Geometry check sheet. Reference: the model listing, model coordinates, mm. A direction names the side the tool comes from. Round coordinates to 2 decimals unless told otherwise and drop trailing zeros. Loops run counter-clockwise (first coordinate to the right, second up) from the corner with the lowest first, then second, coordinate; pieces in that order, holes last. Notation, with made-up numbers: (-16, -18.5) - (35, -18.5) arc R23 cw to (35, 19.5) - close; hole circle Ø11 at (73, 52.25). An arc over 180 degrees is marked (long way). Write item = value, one per line.
```python
from build123d import *

# Parameters (mm, degrees)
BOSS_EXTRU_1_DEPTH      = 200
ENL_V_MAT_EXTRU_1_DEPTH = 274.130005675
SYM_TRIE2_COPY_1_DEPTH  = 200
SYM_TRIE2_COPY_2_DEPTH  = 274.130005675
SYM_TRIE2_COPY_3_DEPTH  = 274.130005675
INTERSECT1_START        = -110
INTERSECT1_DEPTH        = 220


# Read off the part's stored shape, not the designer's step: Intersect1
with BuildPart() as part:
    # Esquisse1 → Boss.-Extru.1 (new body)
    with BuildSketch(Plane.XY):
        Polygon((0, 0), (0, 150), (110, 150), (110, 100), (102.516685226, 87), (102.516685226, 77), (110, 64), (110, 14), (71, 0), align=None)
    boss_extru_1 = extrude(amount=BOSS_EXTRU_1_DEPTH)

    # Esquisse5 → Enlèv. mat.-Extru.1 (cut, symmetric)
    with BuildSketch(Plane(origin=(0, 0, 0), x_dir=(0, 0, -1), z_dir=(1, 0, 0))):
        with BuildLine():
            Line((0, 150), (-200, 150))
            Line((-200, 150), (-200, 100))
            ThreePointArc((-200, 100), (-102.931757397, 135.530032876), (0, 145))
            Line((0, 145), (0, 150))
        make_face()
    enl_v_mat_extru_1 = extrude(amount=ENL_V_MAT_EXTRU_1_DEPTH, both=True, mode=Mode.SUBTRACT)

    # Symétrie1: Boss.-Extru.1, Enlèv. mat.-Extru.1 across plane
    add(boss_extru_1.mirror(Plane.XY))
    add(enl_v_mat_extru_1.mirror(Plane.XY), mode=Mode.SUBTRACT)

    # Symétrie2: Boss.-Extru.1 across plane
    add(boss_extru_1.mirror(Plane(origin=(0, 0, 0), x_dir=(0, 0, 1), z_dir=(1, 0, 0))))

    # Symétrie2 copy 1 sketch → Symétrie2 copy 1 (add)
    with BuildSketch(Plane(origin=(0, 0, 0), x_dir=(-1, 0, 0), z_dir=(0, 0, -1))):
        Polygon((0, 0), (0, 150), (110, 150), (110, 100), (102.516685226, 87), (102.516685226, 77), (110, 64), (110, 14), (71, 0), align=None)
    extrude(amount=SYM_TRIE2_COPY_1_DEPTH)

    # Symétrie2 copy 2 sketch → Symétrie2 copy 2 (cut, symmetric)
    with BuildSketch(Plane.ZY):
        with BuildLine():
            Line((0, 150), (-200, 150))
            Line((-200, 150), (-200, 100))
            ThreePointArc((-200, 100), (-102.931757397, 135.530032876), (0, 145))
            Line((0, 145), (0, 150))
        make_face()
    extrude(amount=SYM_TRIE2_COPY_2_DEPTH, both=True, mode=Mode.SUBTRACT)

    # Symétrie2 copy 3 sketch → Symétrie2 copy 3 (cut, symmetric)
    with BuildSketch(Plane(origin=(0, 0, 0), x_dir=(0, 0, -1), z_dir=(-1, 0, 0))):
        with BuildLine():
            Line((0, -150), (-200, -150))
            Line((-200, -150), (-200, -100))
            ThreePointArc((-200, -100), (-102.931757397, -135.530032876), (0, -145))
            Line((0, -145), (0, -150))
        make_face()
    extrude(amount=SYM_TRIE2_COPY_3_DEPTH, both=True, mode=Mode.SUBTRACT)

    # Intersect1 outline → Intersect1 (cut)
    with BuildSketch(Plane.YZ.offset(INTERSECT1_START)):
        with BuildLine():
            ThreePointArc((100, -200), (110.281899779, -178.766997787), (119.294166687, -156.964775625))
            Line((119.294166687, -156.964775625), (0, -125))
            Line((0, -125), (0, -200))
            Line((0, -200), (100, -200))
        make_face()
        with BuildLine():
            Line((0, 200), (0, 125))
            Line((0, 125), (106.673784722, 186.588138325))
            ThreePointArc((106.673784722, 186.588138325), (103.399684527, 193.325314743), (100, 200))
            Line((100, 200), (0, 200))
        make_face()
    extrude(amount=INTERSECT1_DEPTH, mode=Mode.SUBTRACT)


solid = part.part
```
(1) Mould release check, pull along Y, two halves, no side actions. Record for faces 1 (the cylindrical face through (1.54, 139.845, -80.879)), 2 (the flat face through (-106.2, 70.6, 14.1)), 3 (the flat face through (110, 118, 17)), 4 (the flat face through (-90.773, 7.098, 3.999)): pulls with the +Y half, pulls with the -Y half, needs draft (parallel to the pull), parting line crosses it, or undercut.
Answers follow:
face_1 = pulls with the +Y half
face_2 = undercut
face_3 = needs draft
face_4 = pulls with the -Y half
(2) Gauge pin test, flat ends, axial feed: pin 1 (6 mm diameter, centred on x = 27.5, z = -112.5, fed in from +Y); pin 2 (4 mm diameter, centred on y = 86, z = -36.5, fed in from -X); pin 3 (6 mm diameter, centred on x = 66.5, z = 105.5, fed in from +Y). Record the tip position at first contact, or that the pin passes through.
Answers follow:
pin_1 = 133.99
pin_2 = -103.09
pin_3 = 135.63
(3) Scan lines: L1, parallel to X at y = 98.5, z = -118; L2, parallel to X at y = 67, z = -142.5; L3, parallel to Y at x = 85, z = 170. Record each from-to range of solid material in increasing order. Write a range as [from, to].
Answers follow:
L1 = [-109.14, 109.14]
L2 = [-108.27, 108.27]
L3 = [77.94, 114.09]
(4) Section check C-C (y = 123.5). Enter the section's corners in (x, z).
Answers follow:
outline = (-110, -145.34) - (110, -145.34) - (110, 145.34) - (-110, 145.34) - close
(5) Section check A-A (z = 94). Enter the section's corners in (x, y).
Answers follow:
outline = (-110, 14) - (-71, 0) - (71, 0) - (110, 14) - (110, 64) - (102.52, 77) - (102.52, 87) - (110, 100) - (110, 137.43) - (-110, 137.43) - (-110, 100) - (-102.52, 87) - (-102.52, 77) - (-110, 64) - close
(6) Section check D-D (z = 14). Enter the section's corners in (x, y), then the cut area to 3 significant figures.
Answers follow:
outline = (-110, 14) - (-71, 0) - (71, 0) - (110, 14) - (110, 64) - (102.52, 77) - (102.52, 87) - (110, 100) - (110, 145.28) - (-110, 145.28) - (-110, 100) - (-102.52, 87) - (-102.52, 77) - (-110, 64) - close
area = 31,100 mm²
(7) Set-up check for faces 5 (the flat face through (-106.31, 93.59, 17.81)), 6 (the flat face through (106.2, 70.6, 14.1)), 7 (the flat face through (-1.54, 60.482, -141.206)): record each of +Z, -Z, +X, -X, +Y, -Y from which the full face is reachable in a straight line by a thin tool's end or side.
Answers follow:
face_5 = +Z, -Z, -X
face_6 = +Z, -Z, +X
face_7 = -Z, +X, -X, -Y
(8) Section check B-B (x = 22.5). Enter the section's corners in (y, z).
Answers follow:
outline = (0, -125) - (119.29, -156.96) arc R400 ccw to (145, 0) arc R400 ccw to (106.67, 186.59) - (0, 125) - close
